Check sheet for the modelled part. Datum: model origin and axes. Units: mm. Face numbers are marked on the shaded views. A direction names the side the tool comes from. Round coordinates to 2 decimals unless told otherwise and drop trailing zeros. Order: outer loops, then holes, each group sorted by start corner. A loop starts at its lowest first (then second) coordinate and runs counter-clockwise, first axis right, second up. Notation, with made-up numbers: (40.25, -8.75) -> (88.25, -8.75) arc R22 cw to (88.25, 14.25) -> close; hole circle Ø11 at (71, 26). An arc over 180 degrees is marked (long way). Answer in a Markdown table with one row per item.
from build123d import *

# Parameters (mm, degrees)
EXTRUDE_1_DEPTH     = 90
SKETCH_2_R          = 4
SKETCH_2_R_2        = 1.5
CUT_EXTRUDE_1_DEPTH = 90
FILLET_1_R          = 5


with BuildPart() as part:
    # 草图1 → 凸台-拉伸1 (new body)
    with BuildSketch(Plane.XY):
        Polygon((-14.5, 40), (-14.5, -2), (14.5, -2), (14.5, 40), (12.5, 40), (12.5, 0), (-12.5, 0), (-12.5, 40), align=None)
    extrude(amount=-EXTRUDE_1_DEPTH)

    # 草图2 → 切除-拉伸1 (cut)
    with BuildSketch(Plane(origin=(14.5, 0, 0), x_dir=(0, 0, -1), z_dir=(1, 0, 0))):
        with Locations(Location((79.75, 28, 0), (0, 0, 90))):
            Circle(SKETCH_2_R)
        with Locations(Location((79.75, 35, 0), (0, 0, 90))):
            Circle(SKETCH_2_R_2)
        with Locations(Location((86.75, 28, 0), (0, 0, 90))):
            Circle(SKETCH_2_R_2)
        with Locations(Location((79.75, 21, 0), (0, 0, 90))):
            Circle(SKETCH_2_R_2)
        with Locations(Location((72.75, 28, 0), (0, 0, 90))):
            Circle(SKETCH_2_R_2)
        with Locations(Location((10.25, 21, 0), (0, 0, 90))):
            Circle(SKETCH_2_R_2)
        with Locations(Location((3.25, 28, 0), (0, 0, 90))):
            Circle(SKETCH_2_R_2)
        with Locations(Location((10.25, 35, 0), (0, 0, 90))):
            Circle(SKETCH_2_R_2)
        with Locations(Location((10.25, 28, 0), (0, 0, 90))):
            Circle(SKETCH_2_R)
        with Locations(Location((17.25, 28, 0), (0, 0, 90))):
            Circle(SKETCH_2_R_2)
        with Locations(Location((45, 28, 0), (0, 0, 90))):
            Circle(SKETCH_2_R)
        with Locations(Location((45, 35, 0), (0, 0, 90))):
            Circle(SKETCH_2_R_2)
        with Locations(Location((52, 28, 0), (0, 0, 90))):
            Circle(SKETCH_2_R_2)
        with Locations(Location((45, 21, 0), (0, 0, 90))):
            Circle(SKETCH_2_R_2)
        with Locations(Location((38, 28, 0), (0, 0, 90))):
            Circle(SKETCH_2_R_2)
    extrude(amount=-CUT_EXTRUDE_1_DEPTH, mode=Mode.SUBTRACT)

    # 圆角1
    fillet_1_edges = [part.edges().sort_by_distance(p)[0] for p in [
        (-13.5, 40, 0),
        (13.5, 40, -90),
        (-13.5, 40, -90),
        (13.5, 40, 0),
    ]]
    fillet(fillet_1_edges, radius=FILLET_1_R)


solid = part.part
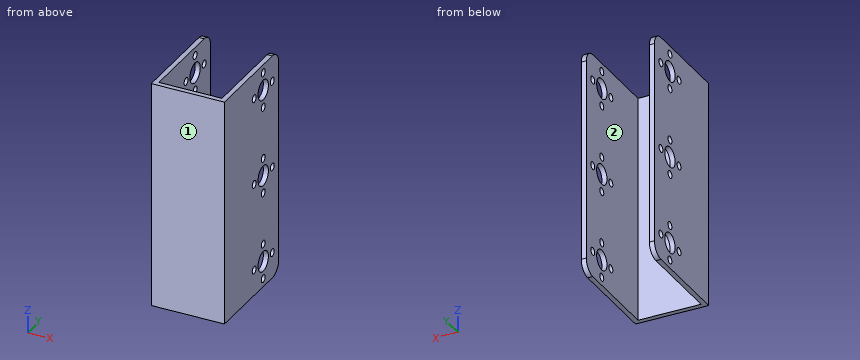
Item 1: Set-up check for the marked faces 1 and 2: record each of +Z, -Z, +X, -X, +Y, -Y from which the full face is reachable in a straight line by a thin tool's end or side.
Result sheet:
| item | result |
|---|---|
| face 1 | +Z, -Z, +X, -X, -Y |
| face 2 | +Z, -Z, +Y |
Item 2: Cross-section at C-C (y = 15). Record the boundary of the cut face in (x, z), and give its area (3 significant figures).
Result sheet:
| item | result |
|---|---|
| outline | (-14.5, -90) -> (-12.5, -90) -> (-12.5, 0) -> (-14.5, 0) -> close; (12.5, -90) -> (14.5, -90) -> (14.5, 0) -> (12.5, 0) -> close |
| area | 360 mm^2 |
Item 3: Scan lines: line 1 (Z direction, x = -13.3, y = 21); line 2 (X direction, y = 14, z = -21.5); line 3 (Y direction, x = 2.25, z = -67.5). Record each from-to range of solid material in increasing order. Write a range as [from, to].
Result sheet:
| item | result |
|---|---|
| line 1 | z = [-90, -81.25], [-78.25, -46.5], [-43.5, -11.75], [-8.75, 0] |
| line 2 | x = [-14.5, -12.5], [12.5, 14.5] |
| line 3 | y = [-2, 0] |
Item 4: Depth check by flat-ended pin: P1, Ø3, axis at x = 9.5, y = 14, coming from the -Z side (3 decimals); P2, Ø3, axis at x = -6, z = -20, coming from the +Y side. Enter the tip coordinate at first touch or a pass-through.
Result sheet:
| item | result |
|---|---|
| P1 | passes through |
| P2 | stops at y = 0 |
Item 5: Cross-section at A-A (y = 21). State how many separate pieces and enclosed holes the cut face has, and give its area (3 significant figures).
Result sheet:
| item | result |
|---|---|
| separate pieces | 8 |
| enclosed holes | 0 |
| area | 324 mm^2 |
Item 6: Cross-section at B-B (z = -38). Record the boundary of the cut face in (x, y).
Result sheet:
| item | result |
|---|---|
| outline | (-14.5, -2) -> (14.5, -2) -> (14.5, 26.5) -> (12.5, 26.5) -> (12.5, 0) -> (-12.5, 0) -> (-12.5, 26.5) -> (-14.5, 26.5) -> close; (-14.5, 29.5) -> (-12.5, 29.5) -> (-12.5, 40) -> (-14.5, 40) -> close; (12.5, 29.5) -> (14.5, 29.5) -> (14.5, 40) -> (12.5, 40) -> close |
Item 7: Cross-section at D-D (z = -22). Record the boundary of the cut face in (x, y), and give its area (3 significant figures).
Result sheet:
| item | result |
|---|---|
| outline | (-14.5, -2) -> (14.5, -2) -> (14.5, 40) -> (12.5, 40) -> (12.5, 0) -> (-12.5, 0) -> (-12.5, 40) -> (-14.5, 40) -> close |
| area | 218 mm^2 |
